Could you check a few things on this drawing? It's one solid part, dimensions in mm from its lowest x, y, z. A direction names the side the tool comes from. Round coordinates to 2 decimals unless told otherwise and drop trailing zeros. Loops run counter-clockwise (first coordinate to the right, second up) from the corner with the lowest first, then second, coordinate; pieces in that order, holes last. Notation, with made-up numbers: M 49,-7 L 67,-7 A28 ccw 67,22 Z; hole C -18.75,79 d5. An arc over 180 degrees is marked long. Answer as a JSON object with one key per item and string values.
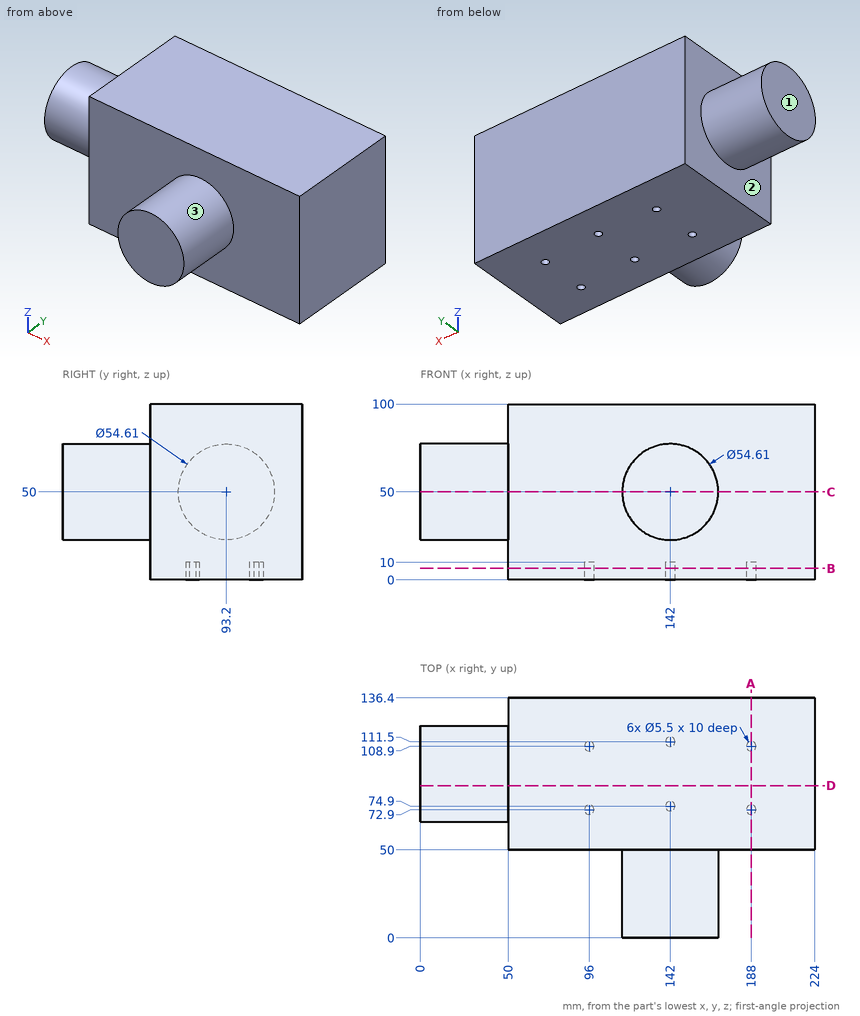
Item 1: On a 3-axis mill with a long thin cutter (end or side, diameter ignored), from which of +Z, -Z, +X, -X, +Y, -Y can I reach the whole of each face in a straight line? I mean the marked faces 1, 2 and 3. Say none if no direction works.
Resolved:
{"face 1": "+Z, -Z, -X, +Y, -Y", "face 2": "-X", "face 3": "-Y"}
Item 2: I want a section at A-A, the plane x = 188. Please give me the cut outline in (y, z), then the cut area to 3 significant figures.
Resolved:
{"outline": "M 50,0 L 70.15,0 L 70.15,10 L 75.65,10 L 75.65,0 L 106.15,0 L 106.15,10 L 111.65,10 L 111.65,0 L 136.4,0 L 136.4,100 L 50,100 Z", "area": "8,530 mm²"}
Item 3: Please list where these lines run through material, in increasing order: probe 1 along Y at (x, z) = (96, 7.25); probe 2 along Y at (x, z) = (142, 7.25); probe 3 along X at (y, z) = (59, 25). Write a range as from..to.
Resolved:
{"probe 1": "50..70.15, 75.65..106.15, 111.65..136.4", "probe 2": "50..72.15, 77.65..108.75, 114.25..136.4", "probe 3": "50..224"}
Item 4: I'm going to push flat-ended pins straight in: pin 1 Ø6 at (x, y) = (96, 74) entering from -Z; pin 2 Ø5 at (x, y) = (188, 108.9) entering from -Z; pin 3 Ø10 at (x, y) = (105.5, 43) entering from +Z; pin 4 Ø4 at (y, z) = (120.5, 86) entering from -X. Where does each tip first touch, or does it pass through?
Resolved:
{"pin 1": "z = 0", "pin 2": "z = 10", "pin 3": "through", "pin 4": "x = 50"}
Item 5: I want a section at B-B, the plane z = 6.5. Please give me the cut outline in (x, y), then the cut area to 3 significant figures.
Resolved:
{"outline": "M 50,50 L 224,50 L 224,136.4 L 50,136.4 Z; hole C 96,72.9 d5.5; hole C 96,108.9 d5.5; hole C 142,74.9 d5.5; hole C 142,111.5 d5.5; hole C 188,72.9 d5.5; hole C 188,108.9 d5.5", "area": "14,900 mm²"}
Item 6: I want a section at D-D, the plane y = 86.5. Please give me the cut outline in (x, z).
Resolved:
{"outline": "M 0,23.53 L 50,23.53 L 50,0 L 224,0 L 224,100 L 50,100 L 50,76.47 L 0,76.47 Z"}
Item 7: I want a section at C-C, the plane z = 50. Please give me the cut outline in (x, y) (3 decimals), then the cut area to 3 significant figures.
Resolved:
{"outline": "M 0,65.895 L 50,65.895 L 50,50 L 114.695,50 L 114.695,0 L 169.305,0 L 169.305,50 L 224,50 L 224,136.4 L 50,136.4 L 50,120.505 L 0,120.505 Z", "area": "20,500 mm²"}
